Can you work these out from the model? Positions are in its coordinate system, mm. Round coordinates to 2 decimals unless told otherwise and drop trailing zeros. Order: outer loops, then holes, each group sorted by start corner. A loop starts at its lowest first (then second) coordinate and runs counter-clockwise, first axis right, second up.
Q1. If we section it at D-D (z = -34): Please give me the cut outline in (x, y).
Q2. If I drill on line 1 (X direction, y = 1.45, z = -34); line 2 (X direction, y = 1.1, z = -22.5); line 3 (X direction, y = 0.75, z = -15.5), over which ranges is the centre line in solid material (lowest first)?
Q3. We'd pull the mould along X, two halves only. Please class faces 1 (the face through (-4, 3, -41)), 2 (the face through (-47.69, 1.48, -48.49)): pulls with the +X half, pulls with the -X half, needs draft (parallel to the pull), parting line crosses it, or undercut.
Q4. If we section it at A-A (z = -24.5): Please give me the cut outline in (x, y).
Q5. Will these pins go through, and if not, where does the flat tip stop? P1, Ø1.4, axis at x = -3, y = 1.5, coming from the +Z side; P2, Ø2, axis at x = -116.25, z = -27.8, coming from the +Y side; P3, Ø1.5, axis at y = 1.5, z = -52, coming from the -X side.
Q6. If we section it at B-B (y = 0.7): Count the separate pieces of the cut face and the enclosed holes in it, plus the area to 3 significant figures.
Q7. If we section it at C-C (x = -98): Please give me the cut outline in (y, z).
from build123d import *

# Parameters (mm, degrees)
ESQUISSE1_R      = 1.25
ESQUISSE1_R_2    = 2.5
EXTRUSION1_DEPTH = 3


with BuildPart() as part:
    # Esquisse1 → Extrusion1 (new body)
    with BuildSketch(Plane(origin=(0, 0, 0), x_dir=(1, 0, 0), z_dir=(0, 1, 0))):
        with BuildLine():
            Line((-119.250326512, 8.795182269), (-113.250326512, 8.795182269))
            Line((-113.250326512, 8.795182269), (-113.250326512, 21.795182269))
            Line((-113.250326512, 21.795182269), (-92.750326512, 21.795182269))
            Line((-92.750326512, 21.795182269), (-92.750326512, 8.795182269))
            Line((-92.750326512, 8.795182269), (-82.750326512, 8.795182269))
            ThreePointArc((-82.750326512, 8.795182269), (-46.875027378, 48.581949451), (-3.600984374, 17.000607921))
            Line((-3.600984374, 17.000607921), (-1.899668651, 17.000607921))
            ThreePointArc((-1.899668651, 17.000607921), (41.374374353, 48.581949451), (77.249673488, 8.795182269))
            Line((77.249673488, 8.795182269), (87.249673488, 8.795182269))
            Line((87.249673488, 8.795182269), (87.249673488, 21.795182269))
            Line((87.249673488, 21.795182269), (107.749673488, 21.795182269))
            Line((107.749673488, 21.795182269), (107.749673488, 8.795182269))
            Line((107.749673488, 8.795182269), (113.749673488, 8.795182269))
            Line((113.749673488, 8.795182269), (113.749673488, 36.099018287))
            Line((113.749673488, 36.099018287), (83.749673488, 36.099018287))
            Line((83.749673488, 36.099018287), (83.749673488, 60.099018287))
            Line((83.749673488, 60.099018287), (-89.250326512, 60.099018287))
            Line((-89.250326512, 60.099018287), (-89.250326512, 36.099018287))
            Line((-89.250326512, 36.099018287), (-119.250326512, 36.099018287))
            Line((-119.250326512, 36.099018287), (-119.250326512, 8.795182269))
        make_face()
        with Locations((110.749673488, 11.795182269)):
            Circle(ESQUISSE1_R, mode=Mode.SUBTRACT)
        with Locations((-2.250326512, 45.599018287)):
            Circle(ESQUISSE1_R_2, mode=Mode.SUBTRACT)
        with Locations((84.249673488, 27.795182269)):
            Circle(ESQUISSE1_R, mode=Mode.SUBTRACT)
        with Locations((110.749673488, 27.795182269)):
            Circle(ESQUISSE1_R, mode=Mode.SUBTRACT)
        with Locations((-80.250326512, 48.795182269)):
            Circle(ESQUISSE1_R_2, mode=Mode.SUBTRACT)
        with Locations((74.749673488, 48.795182269)):
            Circle(ESQUISSE1_R_2, mode=Mode.SUBTRACT)
        with Locations((-116.250326512, 27.795182269)):
            Circle(ESQUISSE1_R, mode=Mode.SUBTRACT)
        with Locations((-89.750326512, 27.795182269)):
            Circle(ESQUISSE1_R, mode=Mode.SUBTRACT)
        with Locations((-89.750326512, 11.795182269)):
            Circle(ESQUISSE1_R, mode=Mode.SUBTRACT)
        with Locations((84.249673488, 11.795182269)):
            Circle(ESQUISSE1_R, mode=Mode.SUBTRACT)
        with Locations((-116.250326512, 11.795182269)):
            Circle(ESQUISSE1_R, mode=Mode.SUBTRACT)
    extrude(amount=EXTRUSION1_DEPTH)


solid = part.part
Solution:
1. outline: (-119.25, 0) - (-73.81, 0) - (-73.81, 3) - (-119.25, 3) - close; (-11.69, 0) - (6.19, 0) - (6.19, 3) - (-11.69, 3) - close; (68.31, 0) - (113.75, 0) - (113.75, 3) - (68.31, 3) - close
2. line 1: x = -119.25 to -73.81, -11.69 to 6.19, 68.31 to 113.75
2. line 2: x = -119.25 to -80.33, -5.17 to -0.33, 74.83 to 113.75
2. line 3: x = -119.25 to -113.25, -92.75 to -82.18, 76.68 to 87.25, 107.75 to 113.75
3. face 1: needs draft
3. face 2: undercut
4. outline: (-119.25, 0) - (-79.54, 0) - (-79.54, 3) - (-119.25, 3) - close; (-5.96, 0) - (0.46, 0) - (0.46, 3) - (-5.96, 3) - close; (74.04, 0) - (113.75, 0) - (113.75, 3) - (74.04, 3) - close
5. P1: stops at z = -17
5. P2: passes through
5. P3: stops at x = -89.25
6. separate pieces: 1
6. enclosed holes: 11
6. area: 4,850 mm2
7. outline: (0, -36.1) - (3, -36.1) - (3, -21.8) - (0, -21.8) - close
